Autodesk Inventor part; units mm, degrees
ref_plane "YZ Plane" through (0, 0, 0) normal (1, 0, 0) x (0, 1, 0)
ref_plane "XZ Plane" through (0, 0, 0) normal (0, 1, 0) x (-1, 0, 0)
ref_plane "XY Plane" through (0, 0, 0) normal (0, 0, 1) x (1, 0, 0)
sketch "Sketch1" plane through (0, 0, 0) normal (0, 0, 1) x (1, 0, 0)
  circle A0 centre (0, 0) radius 16.25
  line L0 (0, 16.25) -> (0, -16.25) construction
  line L1 (-16.25, 0) -> (16.25, 0) construction
  line L2 (-1.5, 16.1806) -> (-1.5, 5.4806)
  line L3 (1.5, 16.1806) -> (1.5, 5.4806)
  line L4 (-1.5, 5.4806) -> (1.5, 5.4806)
  line L5 (-16.1806, 1.5) -> (-5.4806, 1.5)
  line L6 (-5.4806, -1.5) -> (-5.4806, 1.5)
  line L7 (-16.1806, -1.5) -> (-5.4806, -1.5)
  line L8 (-1.5, -16.1806) -> (-1.5, -5.4806)
  line L9 (1.5, -5.4806) -> (-1.5, -5.4806)
  line L10 (1.5, -16.1806) -> (1.5, -5.4806)
  line L11 (16.1806, -1.5) -> (5.4806, -1.5)
  line L12 (5.4806, 1.5) -> (5.4806, -1.5)
  line L13 (16.1806, 1.5) -> (5.4806, 1.5)
  circle A1 centre (0, 0) radius 3.5
  point P0 (0, 5.4806)
  point P1 (-5.4806, 0)
  point P2 (0, -5.4806)
  point P3 (5.4806, 0)
  dimension "d1" = 3
  dimension "d2" = 10.7
  dimension "d5" = 360
  dimension "d7" = 7
  dimension "d12" = 32.5
extrude "Extrusion1" add sketch "Sketch1" along normal mid plane 10 contours L13 L12 L11 A0 L10 L9 L8 L7 L6 L5 L2 L4 L3
properties part number "Rotor"
Part model, mm, in its own coordinate system. A direction names the side the tool comes from. Round coordinates to 2 decimals unless told otherwise and drop trailing zeros. Write each loop counter-clockwise with the first axis right and the second up, starting at its lowest first coordinate (ties: lowest second). Pieces come first, ordered by that corner, then holes.
Item 1: Probe L1, parallel to Y at x = 0, z = 3; L2, parallel to X at y = 11, z = -0.75; L3, parallel to X at y = -0.5, z = -3. List the from-to ranges inside material, lowest first.
Results:
L1: y = -5.48 to -3.5, 3.5 to 5.48
L2: x = -11.96 to -1.5, 1.5 to 11.96
L3: x = -5.48 to -3.46, 3.46 to 5.48
Item 2: Cut at A-A, the plane x = 0. Give the cut face in (y, z).
Results:
outline: (-5.48, -5) - (-3.5, -5) - (-3.5, 5) - (-5.48, 5) - close; (3.5, -5) - (5.48, -5) - (5.48, 5) - (3.5, 5) - close
Item 3: Which spindle directions (+Z, -Z, +X, -X, +Y, -Y) get a long thin tool onto all of the face, cutting with end or side? Do faces 4 (the flat face through (1.5, -11, 0)), 5 (the flat face through (0, 5.481, 0)), 6 (the flat face through (11, -1.5, 0)). Say none if no direction does.
Results:
face 4: +Z, -Z, -Y
face 5: +Z, -Z, +Y
face 6: +Z, -Z, +X
Item 4: Two-plate mould, pull along X, no slides. Class faces 1 (the flat face through (11, 1.5, 0)), 2 (the flat face through (0, -5.481, 0)), 3 (the cylindrical face through (-11.6, 11.38, -0.07)): +X half, -X half, draft (parallel to the pull), parting line (faces both ways), or undercut.
Results:
face 1: draft
face 2: undercut
face 3: -X half
Item 5: Cut at C-C, the plane z = 2. Give the cut face in (x, y).
Results:
outline: (-16.18, -1.5) arc R16.25 ccw to (-1.5, -16.18) - (-1.5, -5.48) - (1.5, -5.48) - (1.5, -16.18) arc R16.25 ccw to (16.18, -1.5) - (5.48, -1.5) - (5.48, 1.5) - (16.18, 1.5) arc R16.25 ccw to (1.5, 16.18) - (1.5, 5.48) - (-1.5, 5.48) - (-1.5, 16.18) arc R16.25 ccw to (-16.18, 1.5) - (-5.48, 1.5) - (-5.48, -1.5) - close; hole circle Ø7 at (0, 0)
Item 6: Drop flat-ended pins along their axis: pin 1 Ø2.5 at (y, z) = (0, -2) entering from -X; pin 2 Ø1.5 at (x, z) = (0.5, -1.5) entering from -Y; pin 3 Ø5 at (y, z) = (12, -2) entering from +X; pin 4 Ø6.5 at (x, y) = (0, 0) entering from -Z. Give the stop position or say it passes through.
Results:
pin 1: stops at x = -5.48
pin 2: stops at y = -5.48
pin 3: stops at x = 13.18
pin 4: passes through
